Can you work these out from the model? Positions are in its coordinate system, mm. Face numbers are marked on the shaded views. A direction names the side the tool comes from. Coordinates: 2 decimals unless noted, no trailing zeros. Write each loop counter-clockwise with the first axis right and the second up, starting at its lowest first coordinate (ties: lowest second). Pieces come first, ordered by that corner, then holes. Notation, with made-up numbers: (-18, 16.25) - (13, 16.25) arc R35 ccw to (13, 50.25) - close; hole circle Ø1 at (-18, 21.5). An arc over 180 degrees is marked (long way). Write each question's results on one line, items separated by ' | '. Start each with the question number.
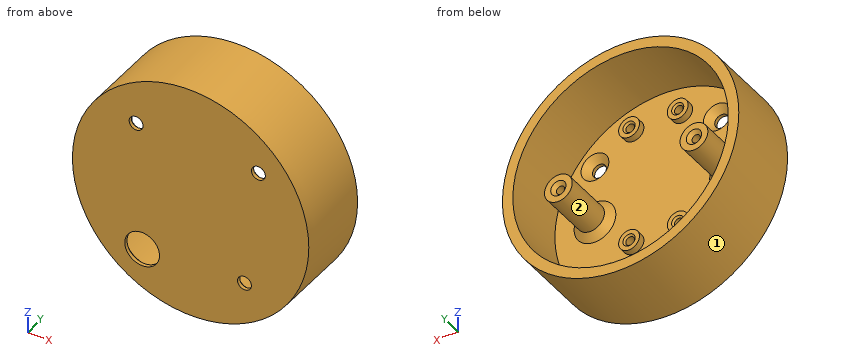
Autodesk Inventor part; units mm, degrees
ref_plane "YZ Plane" through (0, 0, 0) normal (1, 0, 0) x (0, 1, 0)
ref_plane "XZ Plane" through (0, 0, 0) normal (0, 1, 0) x (-1, 0, 0)
ref_plane "XY Plane" through (0, 0, 0) normal (0, 0, 1) x (1, 0, 0)
sketch "Sketch1" plane through (0, 0, 0) normal (0, 1, 0) x (-1, 0, 0)
  circle A0 centre (0, 0) radius 34
  dimension "d0" = 68
extrude "Extrusion1" add sketch "Sketch1" along normal blind 3
sketch "Sketch2" plane through (0, 3, 0) normal (0, 1, 0) x (1, 0, 0)
  circle A0 centre (0, 0) radius 34
  circle A1 centre (0, 0) radius 31
  dimension "d3" = 62
extrude "Extrusion2" add sketch "Sketch2" along normal blind 19
sketch "Sketch3" plane through (0, 3, 0) normal (0, 1, 0) x (1, 0, 0)
  circle A0 centre (0, 0) radius 31
  circle A1 centre (0, 0) radius 19.5
  line L0 (-19.5, 0) -> (19.5, 0)
  circle A2 centre (-19.5, 0) radius 1.2
  circle A3 centre (-19.5, 0) radius 4
  circle A4 centre (19.5, 0) radius 1.2
  circle A5 centre (19.5, 0) radius 4
  dimension "d6" = 39
  dimension "d7" = 2.4
  dimension "d8" = 8
  dimension "d9" = 2.4
  dimension "d10" = 8
extrude "Extrusion3" add sketch "Sketch3" along normal blind 16.5 contours A4 L0 A5 A1 | A1 A5 A4 | A1 A5 L0 A4 | A3 L0 A2 A1 | A1 A2 A3 | A1 A2 L0 A3
chamfer "Chamfer1" distance 2 angle 45 2 edges at (-23.5, 3, 0) (15.5, 3, 0)
sketch "Sketch4" plane through (0, 3, 0) normal (0, 1, 0) x (1, 0, 0)
  circle A0 centre (-13.9417, 19.5241) radius 5
  dimension "d16" = 10
extrude "Extrusion4" cut sketch "Sketch4" against normal blind 14
chamfer "Chamfer2" distance 2 angle 45 1 edges at (-18.9417, 3, -19.5241)
sketch "Sketch5" plane through (0, 3, 0) normal (0, 1, 0) x (1, 0, 0)
  line L0 (-8.5812, 13.9919) -> (11.4188, 13.9919)
  line L1 (11.4188, 13.9919) -> (11.4188, -26.0081)
  line L2 (11.4188, -26.0081) -> (-8.5812, -26.0081)
  line L3 (-8.5812, -26.0081) -> (-8.5812, 13.9919)
  circle A0 centre (-5.5812, 10.9919) radius 1.25
  circle A1 centre (-5.5812, 10.9919) radius 3
  circle A2 centre (8.4188, 10.9919) radius 1.25
  circle A3 centre (8.4188, 10.9919) radius 3
  circle A4 centre (8.4188, -23.0081) radius 1.25
  circle A5 centre (8.4188, -23.0081) radius 3
  circle A6 centre (-5.5812, -23.0081) radius 1.25
  circle A7 centre (-5.5812, -23.0081) radius 3
  dimension "d22" = 20
  dimension "d23" = 40
  dimension "d24" = 2.5
  dimension "d25" = 6
  dimension "d26" = 2.5
  dimension "d27" = 6
  dimension "d28" = 2.5
  dimension "d29" = 6
  dimension "d30" = 2.5
  dimension "d31" = 6
  dimension "d32" = 3
  dimension "d33" = 3
  dimension "d34" = 3
  dimension "d35" = 3
  dimension "d36" = 3
  dimension "d37" = 3
  dimension "d38" = 3
  dimension "d39" = 3
extrude "Extrusion5" add sketch "Sketch5" along normal blind 2 contours A1 | A3 | A7 | A5
sketch "Sketch6" plane through (-5.5812, 3, -10.9919) normal (0, 1, 0) x (1, 0, 0)
  circle A0 centre (0, 0) radius 1.25
  circle A1 centre (0, 0) radius 1.25
  circle A2 centre (14, 0) radius 1.25
  circle A3 centre (14, -34) radius 1.25
  circle A4 centre (0, -34) radius 1.25
  point P0 (5.5812, -10.9919)
extrude "Extrusion6" cut sketch "Sketch6" against normal blind 2
chamfer "Chamfer3" distance 0.5 angle 45 4 edges at (-6.8312, 5, -10.9919) (7.1688, 5, -10.9919) (-6.8312, 5, 23.0081) (7.1688, 5, 23.0081)
chamfer "Chamfer4" distance 1 angle 45 2 edges at (18.3, 19.5, 0) (-20.7, 19.5, 0)
sketch "Sketch7" plane through (0, 3, 0) normal (0, 1, 0) x (1, 0, 0)
  circle A0 centre (-15.6748, -17.735) radius 2
  circle A1 centre (15.4957, 18.0932) radius 2
  circle A2 centre (19.5, -16.6601) radius 2
  dimension "d50" = 4
  dimension "d51" = 4
  dimension "d52" = 4
extrude "Extrusion7" cut sketch "Sketch7" against normal blind 10
chamfer "Chamfer5" distance 2 angle 45 3 edges at (17.5, 3, 16.6601) (-17.6748, 3, 17.735) (13.4957, 3, -18.0932)
properties part number "obudowa - czujnik dymu v2"
Q1. For the marked faces 1 and 2, which set-ups out of +Z, -Z, +X, -X, +Y, -Y let a thin tool reach every point of the face, with its end or its side?
Q2. I'm going to push flat-ended pins straight in: pin 1 Ø12 at (y, z) = (10, -8.5) entering from +X; pin 2 Ø2 at (x, y) = (-21, 10) entering from -Z; pin 3 Ø12 at (x, y) = (-18.5, 3) entering from +Z. Where does each tip first touch, or does it pass through?
Q3. I need wall thicknesses on line 1 along X through (y, z) = (8.75, 0); line 2 along Z through (x, y) = (10, 4.5); line 3 along Z through (x, y) = (-3, 4.75). Which ranges of each line are inside material? Lowest first, please. Write a range as from..to.
Q4. If we section it at A-A (y = 11): Please give me the cut outline in (x, z), then the cut area to 3 significant figures.
Answer list:
1) face 1: +Y, -Y | face 2: +Y
2) pin 1: stops at x = 33.91 | pin 2: stops at z = -27.5 | pin 3: stops at z = 31.62
3) line 1: x = -34..-31, -23.5..-20.7, -18.3..-15.5, 15.5..18.3, 20.7..23.5, 31..34 | line 2: z = -32.5..-29.34, -13.54..-8.44, 20.46..25.56, 29.34..32.5 | line 3: z = -33.87..-30.85, -12.52..-9.46, 21.48..24.54, 30.85..33.87
4) outline: circle Ø68 at (0, 0); circle Ø8 at (-19.5, 0); circle Ø8 at (19.5, 0); hole circle Ø62 at (0, 0); hole circle Ø2.4 at (-19.5, 0); hole circle Ø2.4 at (19.5, 0) | area: 704 mm2
